For this review, use the dimensioned drawing (mm, ordinates from the lowest corner) and the shaded views. Give positions to 0.01 mm unless a question says otherwise; leave off trailing zeros. Order: outer loops, then holes, each group sorted by start corner. A loop starts at its lowest first (then second) coordinate and runs counter-clockwise, first axis right, second up. Notation, with made-up numbers: (37.5, 19) - (67.5, 19) arc R6 ccw to (67.5, 26) - close; hole circle Ø5 at (87, -17.5). An arc over 180 degrees is marked (long way). One line per item, written item: value.
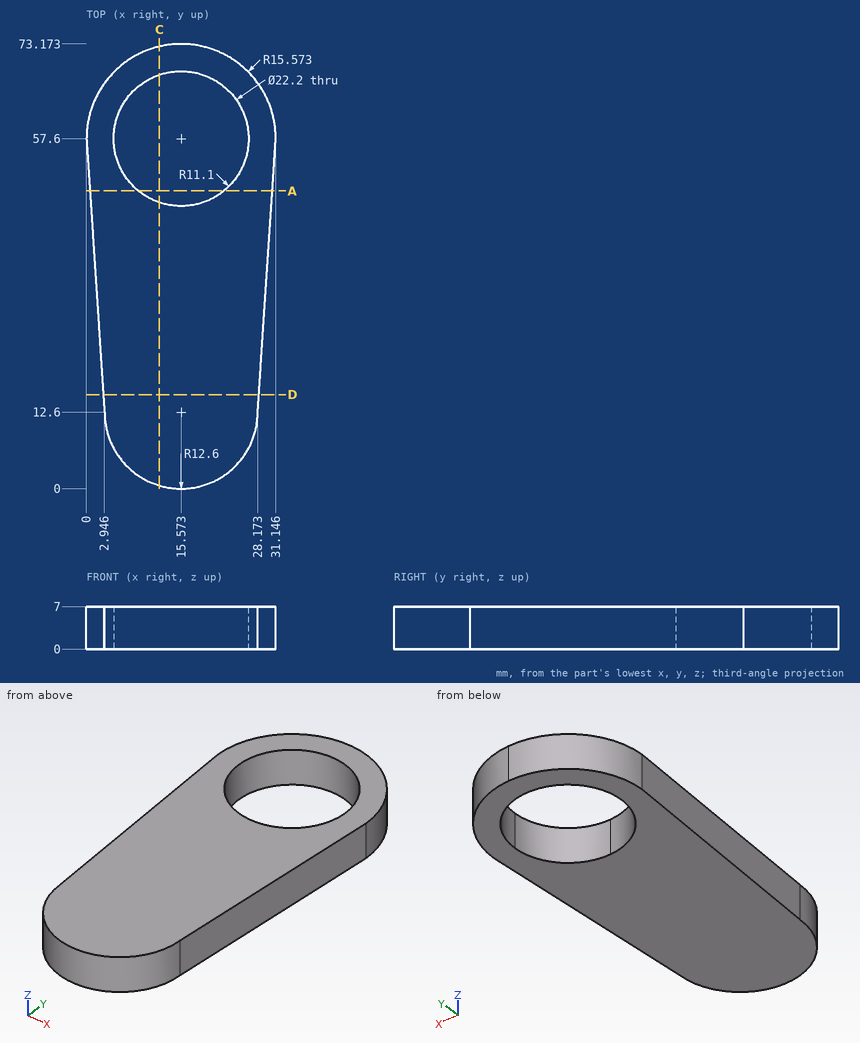
(1) Wall thickness on line 1 (X direction, y = 57.6, z = 2.5); line 2 (Y direction, x = 15, z = 3.75) (1 decimal); line 3 (Y direction, x = 6, z = 2.75) (1 decimal): over which ranges is each line inside the solid? List them lowest first. Write a range as from..to.
Answers below:
line 1: x = 0..4.47, 26.67..31.15
line 2: y = 0..46.5, 68.7..73.2
line 3: y = 4.4..52, 63.2..69.9
(2) Take a section at A-A (y = 49). Write out the cut boundary in (x, z) (1 decimal).
Answers below:
outline: (0.6, 0) - (8.6, 0) - (8.6, 7) - (0.6, 7) - close; (22.6, 0) - (30.6, 0) - (30.6, 7) - (22.6, 7) - close
(3) For P1, Ø1.5, axis at y = 51.5, z = 1, coming from the -X side; P2, Ø2, axis at y = 24, z = 3.5, coming from the +X side; P3, Ø8, axis at x = 15.5, y = 51, coming from the +Z side; P4, Ø1.5, axis at x = 9.5, z = 2.5, coming from the -Y side, all flat-tipped, find the tip position at first contact; note any pin that passes through.
Answers below:
P1: stops at x = 0.35
P2: stops at x = 28.99
P3: passes through
P4: stops at y = 1.18
(4) Take a section at C-C (x = 12). Write out the cut boundary in (y, z).
Answers below:
outline: (0.52, 0) - (47.09, 0) - (47.09, 7) - (0.52, 7) - close; (68.11, 0) - (72.76, 0) - (72.76, 7) - (68.11, 7) - close
(5) Take a section at D-D (y = 15.5). Write out the cut boundary in (x, z) (1 decimal), then the cut area to 3 significant figures.
Answers below:
outline: (2.8, 0) - (28.4, 0) - (28.4, 7) - (2.8, 7) - close
area: 179 mm^2
